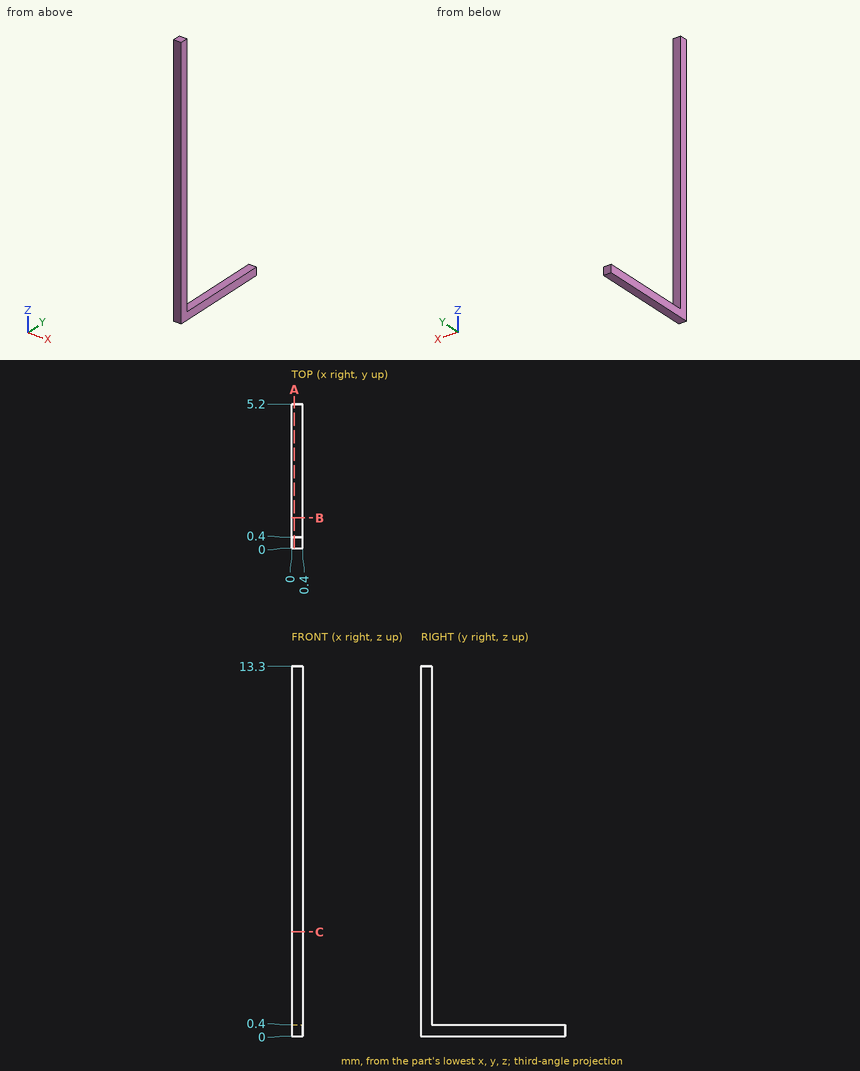
Answer from the drawing. Dimensions are ordinates in mm from the lowest x, y and z of the part. Coordinates: 2 decimals unless noted, no trailing zeros. Loops run counter-clockwise (first coordinate to the right, second up) from the corner with the lowest first, then second, coordinate; pieces in that order, holes last. Notation, with made-up numbers: (-20.5, 37) - (-16.5, 37) arc R21 ccw to (-16.5, 68) - close; hole circle Ø1 at (54, -0.75). An arc over 180 degrees is marked (long way). Answer in a Markdown table with one row per item.
1. Find section A-A, the plane x = 0.1. Write down the section's boundary in (y, z), then the cut area to 3 significant figures.
Conclusion:
| item | result |
|---|---|
| outline | (0, 0) - (5.2, 0) - (5.2, 0.4) - (0.4, 0.4) - (0.4, 13.3) - (0, 13.3) - close |
| area | 7.24 mm² |
2. A straight line is drawn through the part: line 1 (Y direction, x = 0.25, z = 6.25). Find the intervals that lie inside material, in ascending order.
Conclusion:
| item | result |
|---|---|
| line 1 | y = 0 to 0.4 |
3. Find section B-B, the plane y = 1.1. Write down the section's boundary in (x, z), then the cut area to 3 significant figures.
Conclusion:
| item | result |
|---|---|
| outline | (0, 0) - (0.4, 0) - (0.4, 0.4) - (0, 0.4) - close |
| area | 0.160 mm² |
